```python
from build123d import *

# Parameters (mm, degrees)
SKETCH1_W           = 300
SKETCH1_H           = 200
BOSS_EXTRUDE1_DEPTH = 200
CUT_EXTRUDE1_DEPTH  = 375.165738677
SKETCH3_R           = 54
CUT_EXTRUDE2_DEPTH  = 35
CUT_EXTRUDE4_START  = -150
CUT_EXTRUDE4_DEPTH  = 150
CUT_EXTRUDE5_DEPTH  = 20
BOSS_EXTRUDE3_DEPTH = 9.2
SKETCH11_R          = 54
CUT_EXTRUDE6_DEPTH  = 35
CHAMFER1_SIZE       = 40
SKETCH13_R          = 2.5
CUT_EXTRUDE7_DEPTH  = 10
SKETCH14_R          = 2.5
CUT_EXTRUDE8_DEPTH  = 10
CUT_EXTRUDE9_DEPTH  = 105
SKETCH16_W          = 180
SKETCH16_H          = 50
CUT_EXTRUDE10_DEPTH = 15
SKETCH17_W          = 10
SKETCH17_H          = 50
CUT_EXTRUDE11_DEPTH = 5
SKETCH17_3_R        = 1.5
CUT_EXTRUDE12_DEPTH = 10


with BuildPart() as part:
    # Sketch1 → Boss-Extrude1 (new body)
    with BuildSketch(Plane.XY):
        Rectangle(SKETCH1_W, SKETCH1_H)
    extrude(amount=-BOSS_EXTRUDE1_DEPTH)

    # Sketch2 → Cut-Extrude1 (cut, through all)
    with BuildSketch(Plane(origin=(150, 0, 0), x_dir=(0, 0, -1), z_dir=(1, 0, 0))):
        with BuildLine():
            Line((200, 100), (100, 100))
            ThreePointArc((100, 100), (170.710677643, 70.710678595), (200, 1.347e-06))
            Line((200, 1.347e-06), (200, 100))
        make_face()
        with BuildLine():
            Line((200, -100), (200, 1.347e-06))
            ThreePointArc((200, 1.347e-06), (170.710678595, -70.710677643), (100, -100))
            Line((100, -100), (200, -100))
        make_face()
    extrude(amount=-CUT_EXTRUDE1_DEPTH, mode=Mode.SUBTRACT)

    # Sketch3 → Cut-Extrude2 (cut)
    with BuildSketch(Plane(origin=(150, 0, 0), x_dir=(0, 0, -1), z_dir=(1, 0, 0))):
        with Locations((100, 0)):
            Circle(SKETCH3_R)
    extrude(amount=-CUT_EXTRUDE2_DEPTH, mode=Mode.SUBTRACT)

    # Sketch6 → Cut-Extrude4 (cut)
    with BuildSketch(Plane.ZY.offset(150).offset(CUT_EXTRUDE4_START)):
        with BuildLine():
            Line((0, 100), (0, -100))
            Line((0, -100), (-100, -100))
            ThreePointArc((-100, -100), (-200, 0), (-100, 100))
            Line((-100, 100), (0, 100))
        make_face()
    extrude(amount=CUT_EXTRUDE4_DEPTH, mode=Mode.SUBTRACT)

    # Mirror1: part across plane


with BuildPart() as part_1:
    add(part.part)
    add(part.part.mirror(Plane(origin=(0, 0, -100), x_dir=(0, 0, 1), z_dir=(1, 0, 0))))

    # Sketch7 → Cut-Extrude5 (cut)
    with BuildSketch(Plane.XY):
        with BuildLine():
            ThreePointArc((-99.615655403, 75.509742408), (-125, 0), (-99.615655403, -75.509742408))
            ThreePointArc((-99.615655403, -75.509742408), (-78.600607666, -78.402451968), (-75.707898107, -57.38740423))
            ThreePointArc((-75.707898107, -57.38740423), (-95, 0), (-75.707898107, 57.38740423))
            ThreePointArc((-75.707898107, 57.38740423), (-78.600607666, 78.402451968), (-99.615655403, 75.509742408))
        make_face()
        with BuildLine():
            ThreePointArc((75.707898107, 57.38740423), (78.600607666, 78.402451968), (99.615655403, 75.509742408))
            ThreePointArc((99.615655403, 75.509742408), (125, 0), (99.615655403, -75.509742408))
            ThreePointArc((99.615655403, -75.509742408), (78.600607666, -78.402451968), (75.707898107, -57.38740423))
            ThreePointArc((75.707898107, -57.38740423), (95, 0), (75.707898107, 57.38740423))
        make_face()
    extrude(amount=-CUT_EXTRUDE5_DEPTH, mode=Mode.SUBTRACT)

    # Sketch10 → Boss-Extrude3 (add)
    # profile 1 of 2: a face of its own
    with BuildSketch(Plane.XY):
        with BuildLine():
            ThreePointArc((-75.707898107, 57.38740423), (-95, 0), (-75.707898107, -57.38740423))
            ThreePointArc((-75.707898107, -57.38740423), (-78.600607666, -78.402451968), (-99.615655403, -75.509742408))
            ThreePointArc((-99.615655403, -75.509742408), (-125, 0), (-99.615655403, 75.509742408))
            ThreePointArc((-99.615655403, 75.509742408), (-78.600607666, 78.402451968), (-75.707898107, 57.38740423))
        make_face()
        with BuildLine():
            ThreePointArc((-79.692524323, 60.407793927), (-100, 0), (-79.692524323, -60.407793927))
            ThreePointArc((-79.692524323, -60.407793927), (-81.620997362, -74.417825752), (-95.631029187, -72.489352712))
            ThreePointArc((-95.631029187, -72.489352712), (-120, 0), (-95.631029187, 72.489352712))
            ThreePointArc((-95.631029187, 72.489352712), (-81.620997362, 74.417825752), (-79.692524323, 60.407793927))
        make_face(mode=Mode.SUBTRACT)
    # profile 2 of 2: a face of its own
    with BuildSketch(Plane.XY):
        with BuildLine():
            ThreePointArc((75.707898107, -57.38740423), (78.600607666, -78.402451968), (99.615655403, -75.509742408))
            ThreePointArc((99.615655403, -75.509742408), (125, 0), (99.615655403, 75.509742408))
            ThreePointArc((99.615655403, 75.509742408), (78.600607666, 78.402451968), (75.707898107, 57.38740423))
            ThreePointArc((75.707898107, 57.38740423), (95, 0), (75.707898107, -57.38740423))
        make_face()
        with BuildLine():
            ThreePointArc((79.692524323, -60.407793927), (81.620997362, -74.417825752), (95.631029187, -72.489352712))
            ThreePointArc((95.631029187, -72.489352712), (120, 0), (95.631029187, 72.489352712))
            ThreePointArc((95.631029187, 72.489352712), (81.620997362, 74.417825752), (79.692524323, 60.407793927))
            ThreePointArc((79.692524323, 60.407793927), (100, 0), (79.692524323, -60.407793927))
        make_face(mode=Mode.SUBTRACT)
    extrude(amount=-BOSS_EXTRUDE3_DEPTH)

    # Sketch11 → Cut-Extrude6 (cut)
    with BuildSketch(Plane.XY):
        Circle(SKETCH11_R)
    extrude(amount=-CUT_EXTRUDE6_DEPTH, mode=Mode.SUBTRACT)

    # Chamfer1
    chamfer1_edges = [part_1.edges().sort_by_distance(p)[0] for p in [
        (150, 100, -50),
        (150, 0, -200),
        (150, -100, -50),
        (-150, -100, -50),
        (-150, 0, -200),
        (-150, 100, -50),
    ]]
    chamfer(chamfer1_edges, length=CHAMFER1_SIZE)

    # Sketch13 → Cut-Extrude7 (cut)
    with BuildSketch(Plane.ZY.offset(115)):
        with Locations((-100, 30)):
            Circle(SKETCH13_R)
        with Locations((-130, 0)):
            Circle(SKETCH13_R)
        with Locations((-100, -30)):
            Circle(SKETCH13_R)
        with Locations((-70, 0)):
            Circle(SKETCH13_R)
    cut_extrude7 = extrude(amount=-CUT_EXTRUDE7_DEPTH, mode=Mode.SUBTRACT)

    # Mirror2: Cut-Extrude7 across plane
    add(cut_extrude7.mirror(Plane(origin=(0, 0, 0), x_dir=(0, 0, 1), z_dir=(1, 0, 0))), mode=Mode.SUBTRACT)

    # Sketch14 → Cut-Extrude8 (cut)
    with BuildSketch(Plane.XY.offset(-35)):
        with Locations((0, 30)):
            Circle(SKETCH14_R)
        with Locations((-30, 0)):
            Circle(SKETCH14_R)
        with Locations((0, -30)):
            Circle(SKETCH14_R)
        with Locations((30, 0)):
            Circle(SKETCH14_R)
    extrude(amount=-CUT_EXTRUDE8_DEPTH, mode=Mode.SUBTRACT)

    # Sketch15 → Cut-Extrude9 (cut, symmetric)
    with BuildSketch(Plane(origin=(0, 0, 0), x_dir=(0, 0, -1), z_dir=(1, 0, 0))):
        with BuildLine():
            ThreePointArc((100, 90), (190, 0), (100, -90))
            Line((100, -90), (45, -90))
            Line((45, -90), (45, 90))
            Line((45, 90), (100, 90))
        make_face()
    extrude(amount=CUT_EXTRUDE9_DEPTH, both=True, mode=Mode.SUBTRACT)

    # Sketch16 → Cut-Extrude10 (cut)
    with BuildSketch(Plane.XZ.offset(100)):
        with Locations((0, -70)):
            Rectangle(SKETCH16_W, SKETCH16_H)
    extrude(amount=-CUT_EXTRUDE10_DEPTH, mode=Mode.SUBTRACT)

    # Sketch17 → Cut-Extrude11 (cut)
    with BuildSketch(Plane.XZ.offset(100)):
        with Locations((95, -70)):
            Rectangle(SKETCH17_W, SKETCH17_H)
        with Locations((-95, -70)):
            Rectangle(SKETCH17_W, SKETCH17_H)
    extrude(amount=-CUT_EXTRUDE11_DEPTH, mode=Mode.SUBTRACT)

    # Sketch17_3 → Cut-Extrude12 (cut)
    with BuildSketch(Plane.XZ.offset(100)):
        with Locations(Location((-95, -50, 0), (0, 0, 270))):
            Circle(SKETCH17_3_R)
        with Locations(Location((95, -50, 0), (0, 0, 270))):
            Circle(SKETCH17_3_R)
        with Locations(Location((-95, -60, 0), (0, 0, 270))):
            Circle(SKETCH17_3_R)
        with Locations(Location((95, -60, 0), (0, 0, 270))):
            Circle(SKETCH17_3_R)
        with Locations(Location((-95, -70, 0), (0, 0, 270))):
            Circle(SKETCH17_3_R)
        with Locations(Location((95, -70, 0), (0, 0, 270))):
            Circle(SKETCH17_3_R)
        with Locations(Location((-95, -80, 0), (0, 0, 270))):
            Circle(SKETCH17_3_R)
        with Locations(Location((95, -80, 0), (0, 0, 270))):
            Circle(SKETCH17_3_R)
        with Locations(Location((-95, -90, 0), (0, 0, 270))):
            Circle(SKETCH17_3_R)
        with Locations(Location((95, -90, 0), (0, 0, 270))):
            Circle(SKETCH17_3_R)
    extrude(amount=-CUT_EXTRUDE12_DEPTH, mode=Mode.SUBTRACT)


solid = part_1.part
```
Check sheet for the modelled part. Datum: model origin and axes. Units: mm. A direction names the side the tool comes from. Round coordinates to 2 decimals unless told otherwise and drop trailing zeros. Write item = value, one per line. Start each with the question number.
Q1. Depth check by flat-ended pin: P1, Ø15.5, axis at x = 86.5, y = 17, coming from the -Z side; P2, Ø10, axis at x = 84.5, z = -128.5, coming from the -Y side; P3, Ø8, axis at x = -30, y = 0, coming from the +Z side. Enter the tip coordinate at first touch or a pass-through.
Q2. Access from +Z, -Z, +X, -X, +Y, -Y to the whole of each face (thin tool, end or side, straight path). Record for faces 5 (the face through (-119.995, -1.09, -4.536)), 6 (the face through (-99, 1, -20)), 7 (the face through (-97, -95, -70)), 8 (the face through (132.745, 16.22, -151.506)).
Q3. Release check for a two-part mould opening along Y. For faces 1 (the face through (-130, 80, -51)), 2 (the face through (1.47, 1.98, -189.98)), 3 (the face through (-78.87, -78.6, -14.52)), 4 (the face through (35, 46, 0)) record: pulls with the +Y half, pulls with the -Y half, needs draft (parallel to the pull), parting line crosses it, or undercut.
Q4. Thickness scan on L1, parallel to Y at x = 0, z = -37; L2, parallel to X at y = 51, z = -72.5; L3, parallel to X at y = 36.5, z = -19. Record the ranges inside material, lowest first.
Derived:
q1.P1 = -199.57
q1.P2 = -97.2
q1.P3 = -35
q2.face_5 = +Z
q2.face_6 = none
q2.face_7 = -Y
q2.face_8 = +X
q3.face_1 = pulls with the +Y half
q3.face_2 = undercut
q3.face_3 = undercut
q3.face_4 = needs draft
q4.L1 = -100 to -32.5, -27.5 to 27.5, 32.5 to 100
q4.L2 = -150 to -105, 105 to 150
q4.L3 = -150 to -119.55, -87.71 to -39.8, 39.8 to 87.71, 119.55 to 150
